The listing builds one solid part. Answer for the finished solid, in the listing's coordinates (mm). A direction names the side the tool comes from. Give positions to 0.01 mm unless a question says otherwise; leave off trailing zeros. Write each loop counter-clockwise with the first axis right and the second up, starting at its lowest first coordinate (ties: lowest second). Pieces come first, ordered by that corner, then holes. Notation, with made-up numbers: (-31, -15.5) - (14, -15.5) arc R11 cw to (14, -11.5) - close; hole circle Ø6 at (-32, 14.25). An arc over 180 degrees is marked (long way). Answer in a Markdown table with one row per item. Add a question column.
from build123d import *

# Parameters (mm, degrees)
SKETCH1_W           = 50.8
SKETCH1_H           = 41.275
SKETCH1_R           = 2.286
SKETCH1_R_2         = 3.407671893
SKETCH1_R_3         = 4.051699908
SKETCH1_W_2         = 12.7
SKETCH1_H_2         = 3.175
BOSS_EXTRUDE1_DEPTH = 3.175


with BuildPart() as part:
    # Sketch1 → Boss-Extrude1 (new body)
    with BuildSketch(Plane.XY):
        with Locations((25.4, 20.6375)):
            Rectangle(SKETCH1_W, SKETCH1_H)
        with Locations((25.4, 28.575)):
            Circle(SKETCH1_R, mode=Mode.SUBTRACT)
        with Locations((7.98153171, 26.761776277)):
            Circle(SKETCH1_R_2, mode=Mode.SUBTRACT)
        with Locations((32.727276231, 28.575)):
            Circle(SKETCH1_R_3, mode=Mode.SUBTRACT)
        with Locations((12.7, 7.9375)):
            Rectangle(SKETCH1_W_2, SKETCH1_H_2, mode=Mode.SUBTRACT)
        with Locations((38.1, 7.9375)):
            Rectangle(SKETCH1_W_2, SKETCH1_H_2, mode=Mode.SUBTRACT)
    extrude(amount=BOSS_EXTRUDE1_DEPTH)


solid = part.part
1. A tool of negligible diameter and unlimited length cuts with its end or side. For faces 1 (the face through (6.35, 8, 2)), 2 (the face through (50.8, 20, 2)), from which of +Z, -Z, +X, -X, +Y, -Y can it reach the whole face along a straight path? Write none if from no direction.
2. Section D-D (x = 42.5) is taken. Give the vertices of the cut face in (y, z) (3 decimals).
3. Section C-C (z = 2.4) is taken. Give the vertices of the cut face in (x, y) (3 decimals), and give its area (3 significant figures).
4. Straight lines are drawn through the part: L1, parallel to Y at x = 32.5, z = 3.05 (3 decimals); L2, parallel to Y at x = 14.5, z = 0.25 (3 decimals); L3, parallel to Y at x = 6.5, z = 1.55 (3 decimals). For each, find the intervals that lie inside material, in ascending order. Write a range as [from, to].
5. Section B-B (y = 9) is taken. Give the vertices of the cut face in (x, z) (3 decimals), and give its area (3 significant figures).
6. The mould has two halves that part along X. Classify faces 3 (the face through (9.813, 29.635, 1.565)), 4 (the face through (25, 21, 0)), 5 (the face through (0, 20, 2)): +X half, -X half, draft (parallel to the pull), parting line (faces both ways), or undercut.
7. Section A-A (x = 25.4) is taken. Give the vertices of the cut face in (y, z) (3 decimals), and give its area (3 significant figures).
Geometry check:
| question | item | result |
|---|---|---|
| 1 | face 1 | +Z, -Z |
| 1 | face 2 | +Z, -Z, +X, +Y, -Y |
| 2 | outline | (0, 0) - (6.35, 0) - (6.35, 3.175) - (0, 3.175) - close; (9.525, 0) - (41.275, 0) - (41.275, 3.175) - (9.525, 3.175) - close |
| 3 | outline | (0, 0) - (50.8, 0) - (50.8, 41.275) - (0, 41.275) - close; hole circle Ø6.815 at (7.982, 26.762); hole (6.35, 6.35) - (19.05, 6.35) - (19.05, 9.525) - (6.35, 9.525) - close; hole circle Ø4.572 at (25.4, 28.575); hole circle Ø8.103 at (32.727, 28.575); hole (31.75, 6.35) - (44.45, 6.35) - (44.45, 9.525) - (31.75, 9.525) - close |
| 3 | area | 1,910 mm² |
| 4 | L1 | [0, 6.35], [9.525, 24.53], [32.62, 41.275] |
| 4 | L2 | [0, 6.35], [9.525, 41.275] |
| 4 | L3 | [0, 6.35], [9.525, 23.693], [29.831, 41.275] |
| 5 | outline | (0, 0) - (6.35, 0) - (6.35, 3.175) - (0, 3.175) - close; (19.05, 0) - (31.75, 0) - (31.75, 3.175) - (19.05, 3.175) - close; (44.45, 0) - (50.8, 0) - (50.8, 3.175) - (44.45, 3.175) - close |
| 5 | area | 80.6 mm² |
| 6 | face 3 | undercut |
| 6 | face 4 | draft |
| 6 | face 5 | -X half |
| 7 | outline | (0, 0) - (26.289, 0) - (26.289, 3.175) - (0, 3.175) - close; (30.861, 0) - (41.275, 0) - (41.275, 3.175) - (30.861, 3.175) - close |
| 7 | area | 117 mm² |
